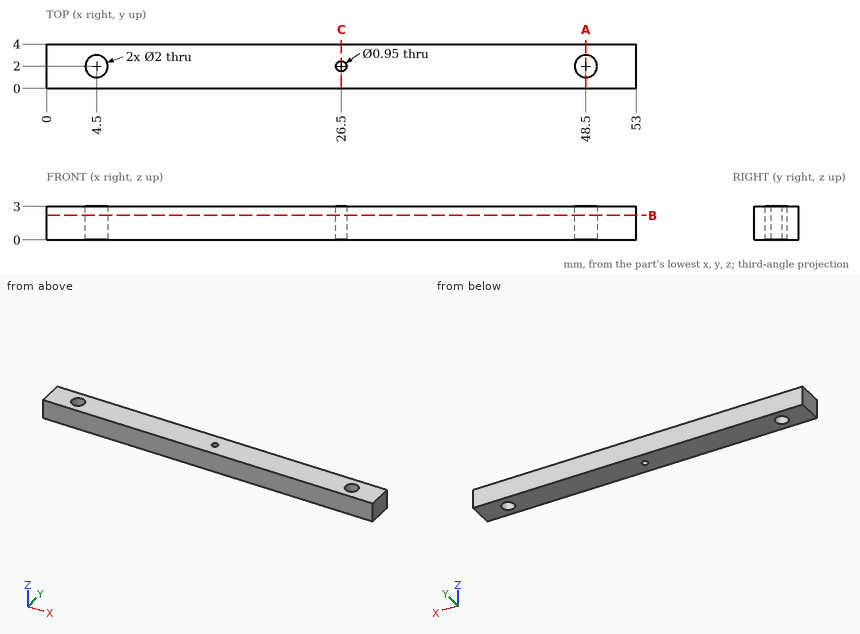
Answer from the drawing. Dimensions are ordinates in mm from the lowest x, y and z of the part. Give positions to 0.01 mm unless a question says otherwise; leave off trailing zeros. Loops run counter-clockwise (first coordinate to the right, second up) from the corner with the lowest first, then second, coordinate; pieces in that order, holes last. Notation, with made-up numbers: (45.25, 51) - (61.25, 51) arc R17 ccw to (61.25, 76) - close; hole circle Ø9 at (50.25, -19). An arc over 180 degrees is marked (long way). Write each question's results on one line, items separated by ' | '.
1. Find section A-A, the plane x = 48.5. Write down the section's boundary in (y, z).
Resolved:
outline: (0, 0) - (1, 0) - (1, 3) - (0, 3) - close; (3, 0) - (4, 0) - (4, 3) - (3, 3) - close
2. Find section C-C, the plane x = 26.5. Write down the section's boundary in (y, z) (3 decimals), then the cut area to 3 significant figures.
Resolved:
outline: (0, 0) - (1.525, 0) - (1.525, 3) - (0, 3) - close; (2.475, 0) - (4, 0) - (4, 3) - (2.475, 3) - close | area: 9.15 mm^2
3. Find section B-B, the plane z = 2.2. Write down the section's boundary in (x, y) (3 decimals).
Resolved:
outline: (0, 0) - (53, 0) - (53, 4) - (0, 4) - close; hole circle Ø2 at (4.5, 2); hole circle Ø0.95 at (26.5, 2); hole circle Ø2 at (48.5, 2)
4. Consider probe 1 along Y at (x, z) = (26.5, 0.7) (3 decimals); probe 2 along X at (y, z) = (2.35, 2.7); probe 3 along Y at (x, z) = (4.5, 0.8). Determine where each line is inside the solid, lowest interval first. Write a range as from..to.
Resolved:
probe 1: y = 0..1.525, 2.475..4 | probe 2: x = 0..3.56, 5.44..26.18, 26.82..47.56, 49.44..53 | probe 3: y = 0..1, 3..4
